Autodesk Inventor part; units mm, degrees
ref_plane "YZ Plane" through (0, 0, 0) normal (1, 0, 0) x (0, 1, 0)
ref_plane "XZ Plane" through (0, 0, 0) normal (0, 1, 0) x (-1, 0, 0)
ref_plane "XY Plane" through (0, 0, 0) normal (0, 0, 1) x (1, 0, 0)
sketch "Sketch5" plane through (0, 0, 0) normal (0, 0, 1) x (1, 0, 0)
  line L0 (-121.5, 134) -> (121.5, 134)
  line L1 (121.5, 134) -> (121.5, -134)
  line L2 (121.5, -134) -> (-121.5, -134)
  line L3 (-121.5, -134) -> (-121.5, 134)
  point P0 (0, 0)
  point P1 (0, 134)
  point P2 (121.5, 0)
  dimension "d8" = 243
  dimension "d43" = 268
extrude "Extrusion5" add sketch "Sketch5" along normal blind 10
sketch "Sketch6" plane through (0, 0, 10) normal (0, 0, 1) x (1, 0, 0)
  line L0 (-52.5, 55) -> (52.5, 55)
  line L1 (52.5, 55) -> (52.5, -55)
  line L2 (52.5, -55) -> (-52.5, -55)
  line L3 (-52.5, -55) -> (-52.5, 55)
  arc A0 (46.5, -55) -> (52.5, -55) centre (49.5, -55) ccw
  arc A1 (-52.5, -55) -> (-46.5, -55) centre (-49.5, -55) ccw
  arc A2 (-46.5, 55) -> (-52.5, 55) centre (-49.5, 55) ccw
  arc A3 (52.5, 55) -> (46.5, 55) centre (49.5, 55) ccw
  point P0 (0, 0)
  point P1 (-52.5, 0)
  point P2 (0, -55)
  dimension "d12" = 105
  dimension "d13" = 110
  dimension "d108" = 6
extrude "Extrusion6" cut sketch "Sketch6" against normal through all
sketch "Sketch7" plane through (0, 0, 10) normal (0, 0, 1) x (1, 0, 0)
  line L0 (121.5, 134) -> (-121.5, 134)
  line L1 (121.5, -134) -> (121.5, 134)
  line L2 (121.5, 70) -> (67.5, 70)
  line L3 (67.5, 70) -> (67.5, 134)
  line L4 (67.5, 134) -> (121.5, 134)
  line L5 (121.5, 134) -> (121.5, 70)
  line L6 (0, 0) -> (0, 14.6341) construction
  circle A0 centre (27.5, 125) radius 4.5
  circle A1 centre (-27.5, 125) radius 4.5
  line L7 (-121.5, 70) -> (-67.5, 70)
  line L8 (-67.5, 70) -> (-67.5, 134)
  line L9 (-67.5, 134) -> (-121.5, 134)
  line L10 (-121.5, 134) -> (-121.5, 70)
  line L11 (121.5, -134) -> (67.5, -134)
  line L12 (67.5, -134) -> (67.5, -84)
  line L13 (67.5, -84) -> (121.5, -84)
  line L14 (121.5, -84) -> (121.5, -134)
  circle A2 centre (27.5, -78) radius 4.5
  circle A3 centre (-27.5, -78) radius 4.5
  line L15 (-121.5, -134) -> (-67.5, -134)
  line L16 (-67.5, -134) -> (-67.5, -84)
  line L17 (-67.5, -84) -> (-121.5, -84)
  line L18 (-121.5, -84) -> (-121.5, -134)
  line L19 (-121.5, -134) -> (121.5, -134)
  point P0 (-121.5, -69)
  dimension "d23" = 64
  dimension "d63" = 67.5
  dimension "d88" = 50
  dimension "d89" = 54
  dimension "d90" = 54
extrude "Extrusion7" cut sketch "Sketch7" against normal through all contours L1 L2 L3 L0 | L15 L18 L17 L16 | L1 L11 L12 L13 | L8 L7 L10 L0
sketch "Sketch8" plane through (0, 0, 10) normal (0, 0, 1) x (1, 0, 0)
  line L0 (0, 0) -> (0, 14.6341) construction
  circle A0 centre (27.5, -125) radius 4.5
  circle A1 centre (-27.5, -125) radius 4.5
  circle A2 centre (27.5, 125) radius 4.5
  circle A3 centre (-27.5, 125) radius 4.5
  circle A4 centre (76.5, -70) radius 4.5
  circle A5 centre (-76.5, -70) radius 4.5
  circle A6 centre (104.5, -70) radius 4.5
  circle A7 centre (-104.5, -70) radius 4.5
  dimension "d28" = 55
  dimension "d29" = 27.5
  dimension "d30" = 9
  dimension "d31" = 250
  dimension "d41" = 55
  dimension "d48" = 153
  dimension "d49" = 76.5
  dimension "d50" = 55
  dimension "d51" = 125
  dimension "d53" = 28
  dimension "d54" = 28
hole "Hole1" at (27.5, -125, 10) at (-27.5, -125, 10) at (-27.5, 125, 10) at (27.5, 125, 10) at (104.5, -70, 10) at (76.5, -70, 10) at (-76.5, -70, 10) at (-104.5, -70, 10) direction (0, 0, -1) diameter 5.5 end through all counterbore diameter 10 counterbore depth 5.5
chamfer "Chamfer1" distance 15 angle 45 4 edges at (-67.5, 134, 5) (67.5, 134, 5) (67.5, -134, 5) (-67.5, -134, 5)
fillet "Fillet2" radius 4 4 edges at (67.5, 70, 5) (-67.5, 70, 5) (67.5, -84, 5) (-67.5, -84, 5)
sketch "Sketch10" plane through (0, 0, 10) normal (0, 0, 1) x (1, 0, 0)
  line L0 (121.5, -84) -> (121.5, 70)
  line L1 (118.5, -50) -> (56, -50)
  line L2 (56, -50) -> (56, 134)
  line L3 (56, 134) -> (118.5, 134)
  line L4 (118.5, 134) -> (118.5, -50)
  line L5 (0, 0) -> (0, -20.3736) construction
  line L6 (-118.5, -50) -> (-56, -50)
  line L7 (-56, -50) -> (-56, 134)
  line L8 (-56, 134) -> (-118.5, 134)
  line L9 (-118.5, 134) -> (-118.5, -50)
  line L10 (52.5, 134) -> (-52.5, 134)
  arc A0 (112.5, -50) -> (118.5, -50) centre (115.5, -50) ccw
  arc A1 (56, -50) -> (62, -50) centre (59, -50) ccw
  circle A2 centre (-115.5, -50) radius 3
  circle A3 centre (-59, -50) radius 3
  point P0 (-112.5, -50)
  dimension "d57" = 62.5
  dimension "d59" = 56
  dimension "d60" = 3
  dimension "d101" = 50
  dimension "d107" = 6
extrude "Extrusion8" cut sketch "Sketch10" against normal blind 6.3
sketch "Sketch11" plane through (0, 0, 3.7) normal (0, 0, 1) x (1, 0, 0)
  line L0 (56, -50) -> (56, 130.5)
  line L1 (118.5, -50) -> (56, -50)
  circle A0 centre (102.75, -30) radius 2
  circle A1 centre (71.75, -30) radius 2
  circle A2 centre (102.75, 30) radius 2
  circle A3 centre (71.75, 30) radius 2
  line L2 (0, 0) -> (0, -13.697) construction
  circle A4 centre (-102.75, -30) radius 2
  circle A5 centre (-71.75, -30) radius 2
  circle A6 centre (-102.75, 30) radius 2
  circle A7 centre (-71.75, 30) radius 2
  point P0 (57.5, 50)
  point P1 (56, 130.5)
  dimension "d65" = 60
  dimension "d66" = 20
  dimension "d67" = 31
  dimension "d68" = 15.75
  dimension "d69" = 4
hole "Hole2" at (102.75, -30, 3.7) at (71.75, -30, 3.7) at (71.75, 30, 3.7) at (102.75, 30, 3.7) at (-71.75, 30, 3.7) at (-102.75, 30, 3.7) at (-102.75, -30, 3.7) at (-71.75, -30, 3.7) direction (0, 0, -1) diameter 3.242 end through all
sketch "Sketch12" plane through (0, 0, 3.7) normal (0, 0, 1) x (1, 0, 0)
  line L0 (121.5, 70) -> (71.5, 70)
  circle A0 centre (106, 62.5) radius 3
  line L1 (0, 0) -> (0, 4.9934) construction
  circle A1 centre (-106, 62.5) radius 3
  circle A2 centre (67.5, 62.5) radius 3
  line L2 (-52.5, -55) -> (-52.5, 55)
  line L3 (46.5, -55) -> (-46.5, -55)
  circle A3 centre (-67.5, 62.5) radius 3
  point P0 (121.5, -134)
  point P1 (-52.5, 0)
  point P2 (0, -55)
  dimension "d78" = 7.5
  dimension "d80" = 6
  dimension "d98" = 106
  dimension "d99" = 106
  dimension "d105" = 6
  dimension "d106" = 38.5
hole "Hole3" at (106, 62.5, 3.7) at (-106, 62.5, 3.7) at (67.5, 62.5, 3.7) at (-67.5, 62.5, 3.7) direction (0, 0, -1) diameter 5.5 end through all countersink diameter 11 countersink angle 90
chamfer "Chamfer5" distance 15 angle 45 2 edges at (121.5, -84, 5) (-121.5, -84, 5)
chamfer "Chamfer6" distance 3 angle 45 2 edges at (120, 70, 10) (-120, 70, 10)
equation "\"d90\" = d89"
equation "\"d29\" = 0.5 * d28"
properties part number "BC-10021" material "Alumínio 7075"
Can you work these out from the model? Positions are in its coordinate system, mm. A direction names the side the tool comes from. Round coordinates to 2 decimals unless told otherwise and drop trailing zeros. Loops run counter-clockwise (first coordinate to the right, second up) from the corner with the lowest first, then second, coordinate; pieces in that order, holes last. Notation, with made-up numbers: M 55,13 L 94,13 A23 cw 94,52 Z; hole C 23.5,-31.75 d5. An arc over 180 degrees is marked long. Answer as a JSON object with one key per item and string values. Group by question number.
Q1. Imagine slicing it at A-A, the plane x = 42.5. Please give me the cut outline in (y, z), then the cut area to 3 significant figures.
Q2. Please list where these lines run through material, in increasing order: L1, parallel to X at y = 125, z = 5.8; L2, parallel to X at y = -20, z = 4; L3, parallel to X at y = -30, z = 1.7.
Q3. We'd pull the mould along X, two halves only. Please class faces 6 (the cylindrical face through (-76.621, -67.253, 2.218)), 7 (the flat face through (58.4, 128.1, 2.7)), 8 (the flat face through (-2, -58, 10)): +X half, -X half, draft (parallel to the pull), parting line (faces both ways), or undercut.
Q4. Imagine slicing it at B-B, the plane y = -9. Please give me the cut outline in (x, z), then the cut area to 4 significant figures.
Q5. On a 3-axis mill with a long thin cutter (end or side, diameter ignored), from which of +Z, -Z, +X, -X, +Y, -Y can I reach the whole of each face in a straight line? I mean faces 1 (the flat face through (97, 70, 2)), 2 (the flat face through (-97, 70, 2)), 3 (the flat face through (1, -55, 5)), 4 (the cylindrical face through (-115.6, -53, 6.9)), 5 (the flat face through (79, -72, 4.5)). Say none if no direction works.
Q6. Will these pins go through, and if not, where does the flat tip stop? pin 1 (2 mm diameter, centred on x = -101, z = 4, fed in from +Y); pin 2 (3 mm diameter, centred on x = 71.75, y = -30, fed in from -Z); pin 3 (3 mm diameter, centred on x = -28, y = 127.5, fed in from +Z); pin 4 (3 mm diameter, centred on x = -91, z = 7.5, fed in from +Y).
Findings:
{
 "1": {"outline": "M -134,0 L -55,0 L -55,10 L -134,10 Z; M 55,0 L 134,0 L 134,10 L 55,10 Z", "area": "1,580 mm2"},
 "2": {"L1": "x = -56 to -32.5, -22.5 to 22.5, 32.5 to 56", "L2": "x = -121.5 to -118.5, -56 to -52.5, 52.5 to 56, 118.5 to 121.5", "L3": "x = -121.5 to -104.37, -101.13 to -73.37, -70.13 to -52.5, 52.5 to 70.13, 73.37 to 101.13, 104.37 to 121.5"},
 "3": {"face 6": "undercut", "face 7": "+X half", "face 8": "draft"},
 "4": {"outline": "M -121.5,0 L -52.5,0 L -52.5,10 L -56,10 L -56,3.7 L -118.5,3.7 L -118.5,10 L -121.5,10 Z; M 52.5,0 L 121.5,0 L 121.5,10 L 118.5,10 L 118.5,3.7 L 56,3.7 L 56,10 L 52.5,10 Z", "area": "592.5 mm2"},
 "5": {"face 1": "+Z, -Z, +X, +Y", "face 2": "+Z, -Z, -X, +Y", "face 3": "+Z, -Z", "face 4": "+Z, +Y", "face 5": "+Z"},
 "6": {"pin 1": "stops at y = 70", "pin 2": "passes through", "pin 3": "stops at z = 4.5", "pin 4": "stops at y = -50"}
}
